```python
from build123d import *

# Parameters (mm, degrees)
F1_DEPTH = 9.4869
F2_R     = 3.937
F3_DEPTH = 5.2451
F4_R     = 2.413
F5_DEPTH = 4.2428


with BuildPart() as f1:
    # F0 (on Top) → F1 (new body)
    with BuildSketch(Plane.XY):
        with BuildLine():
            Line((21.283937, 4.7371), (-21.283937, 4.7371))
            ThreePointArc((-21.283937, 4.7371), (-25.4, 0), (-21.283937, -4.7371))
            Line((-21.283937, -4.7371), (21.283937, -4.7371))
            ThreePointArc((21.283937, -4.7371), (25.4, 0), (21.283937, 4.7371))
        make_face()
    extrude(amount=F1_DEPTH)

    # F2 (on face) → F3 (cut)
    with BuildSketch(Plane(origin=(0, 0, 0), x_dir=(1, 0, 0), z_dir=(0, 0, -1))):
        Circle(F2_R)
    extrude(amount=-F3_DEPTH, mode=Mode.SUBTRACT)

    # F4 (on face) → F5 (cut, through all)
    with BuildSketch(Plane(origin=(0, 0, 5.2451), x_dir=(1, 0, 0), z_dir=(0, 0, -1))):
        Circle(F4_R)
    extrude(amount=-F5_DEPTH, mode=Mode.SUBTRACT)


solid = f1.part
```
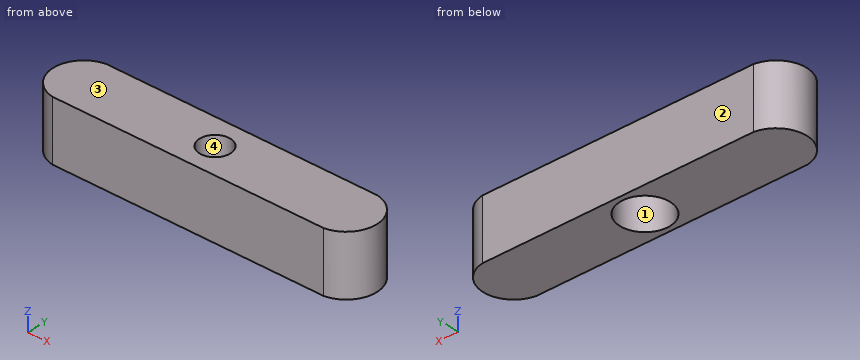
The listing builds one solid part. Answer for the finished solid, in the listing's coordinates (mm). Face numbers are marked on the shaded views. Give positions to 0.01 mm unless a question says otherwise; leave off trailing zeros. Loops run counter-clockwise (first coordinate to the right, second up) from the corner with the lowest first, then second, coordinate; pieces in that order, holes last. Notation, with made-up numbers: (57, 25.25) - (97, 25.25) arc R25 cw to (97, 60.25) - close; hole circle Ø7 at (-4, 82.5). An arc over 180 degrees is marked (long way). Return JSON: item names as keys, results as strings. Group by question number.
1. Find section D-D (z = 3.75). Write down the section's boundary in (x, y).
2. Find section C-C (z = 5.75). Write down the section's boundary in (x, y).
3. Straight lines are drawn through the part: line 1 (Y direction, x = 0, z = 2.9); line 2 (Y direction, x = 0, z = 7.2); line 3 (X direction, y = 0.25, z = 5). For each, find the intervals that lie inside material, in ascending order. Write a range as [from, to].
4. Determine the mould class of the marked faces 1, 2, 3 and 4 for opening direction Y: pulls with the +Y half, pulls with the -Y half, needs draft (parallel to the pull), parting line crosses it, or undercut.
5. Find section B-B (y = 0). Write down the section's boundary in (x, z), then the cut area to 3 significant figures.
6. Find section A-A (x = 0). Write down the section's boundary in (y, z), then the cut area to 3 significant figures.
Verdict:
{
 "1": {"outline": "(-21.28, -4.74) - (21.28, -4.74) arc R4.78 ccw to (21.28, 4.74) - (-21.28, 4.74) arc R4.78 ccw to start; hole circle Ø7.87 at (0, 0)"},
 "2": {"outline": "(-21.28, -4.74) - (21.28, -4.74) arc R4.78 ccw to (21.28, 4.74) - (-21.28, 4.74) arc R4.78 ccw to start; hole circle Ø4.83 at (0, 0)"},
 "3": {"line 1": "y = [-4.74, -3.94], [3.94, 4.74]", "line 2": "y = [-4.74, -2.41], [2.41, 4.74]", "line 3": "x = [-25.39, -3.93], [3.93, 25.39]"},
 "4": {"face 1": "undercut", "face 2": "pulls with the +Y half", "face 3": "needs draft", "face 4": "undercut"},
 "5": {"outline": "(-25.4, 0) - (-3.94, 0) - (-3.94, 5.25) - (-2.41, 5.25) - (-2.41, 9.49) - (-25.4, 9.49) - close; (2.41, 5.25) - (3.94, 5.25) - (3.94, 0) - (25.4, 0) - (25.4, 9.49) - (2.41, 9.49) - close", "area": "420 mm^2"},
 "6": {"outline": "(-4.74, 0) - (-3.94, 0) - (-3.94, 5.25) - (-2.41, 5.25) - (-2.41, 9.49) - (-4.74, 9.49) - close; (2.41, 5.25) - (3.94, 5.25) - (3.94, 0) - (4.74, 0) - (4.74, 9.49) - (2.41, 9.49) - close", "area": "28.1 mm^2"}
}
